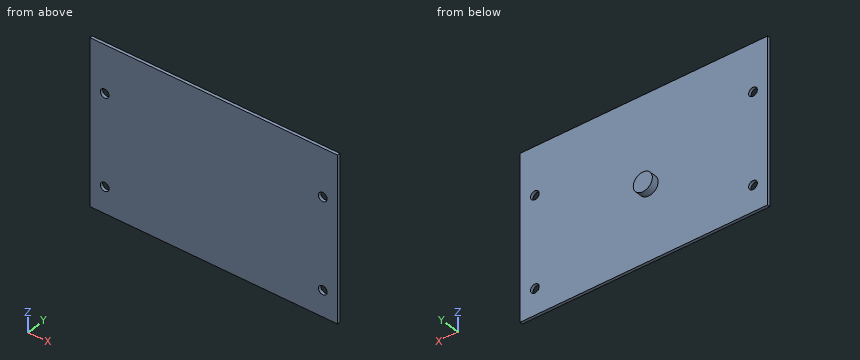
```python
from build123d import *

# Parameters (mm, degrees)
SKETCH1_W           = 85.09
SKETCH1_H           = 56.134
SKETCH1_R           = 1.5
BOSS_EXTRUDE1_DEPTH = 1
SKETCH2_R           = 3.283223987
BOSS_EXTRUDE2_DEPTH = 2.5


with BuildPart() as part:
    # Sketch1 → Boss-Extrude1 (new body)
    with BuildSketch(Plane(origin=(0, 0, 0), x_dir=(1, 0, 0), z_dir=(0, 1, 0))):
        with Locations((42.545, 28.067)):
            Rectangle(SKETCH1_W, SKETCH1_H)
        with Locations(Location((5.01, 47.244, 0), (0, 0, 270))):
            Circle(SKETCH1_R, mode=Mode.SUBTRACT)
        with Locations(Location((80.01, 47.244, 0), (0, 0, 270))):
            Circle(SKETCH1_R, mode=Mode.SUBTRACT)
        with Locations(Location((5.01, 16.244, 0), (0, 0, 270))):
            Circle(SKETCH1_R, mode=Mode.SUBTRACT)
        with Locations(Location((80.01, 16.244, 0), (0, 0, 270))):
            Circle(SKETCH1_R, mode=Mode.SUBTRACT)
    extrude(amount=BOSS_EXTRUDE1_DEPTH)

    # Sketch2 → Boss-Extrude2 (add)
    with BuildSketch(Plane(origin=(0, 1, 0), x_dir=(1, 0, 0), z_dir=(0, 1, 0))):
        with Locations(Location((40.898145706, 31.154537448, 0), (0, 0, 90))):
            Circle(SKETCH2_R)
    extrude(amount=BOSS_EXTRUDE2_DEPTH)


solid = part.part
```
Input: part model. Units: mm. Frame: model coordinates. Coordinates: 2 decimals unless noted, no trailing zeros. Order: outer loops, then holes, each group sorted by start corner. A loop starts at its lowest first (then second) coordinate and runs counter-clockwise, first axis right, second up. Notation, with made-up numbers: (-5, 47.25) - (-1, 47.25) arc R15 cw to (-1, 62.25) - close; hole circle Ø1 at (-13, 35). An arc over 180 degrees is marked (long way). Return JSON: item names as keys, results as strings.
Q1. Ray query, probe 1 along Z at (x, y) = (80.01, 0.45); probe 2 along Z at (x, y) = (6, 0.5); probe 3 along Y at (x, z) = (25, -48). Return the intervals inside material, ascending.
The answers:
{"probe 1": "z = -56.13 to -48.74, -45.74 to -17.74, -14.74 to 0", "probe 2": "z = -56.13 to -48.37, -46.12 to -17.37, -15.12 to 0", "probe 3": "y = 0 to 1"}
Q2. Cut plane A-A (x = 5.01). Return loops of the section in (y, z).
The answers:
{"outline": "(0, -56.13) - (1, -56.13) - (1, -48.74) - (0, -48.74) - close; (0, -45.74) - (1, -45.74) - (1, -17.74) - (0, -17.74) - close; (0, -14.74) - (1, -14.74) - (1, 0) - (0, 0) - close"}
Q3. Cut plane D-D (y = 1.95). Return loops of the section in (x, z).
The answers:
{"outline": "circle Ø6.57 at (40.9, -31.15)"}
Q4. First-contact query: pin 1 (4 mm diameter, centred on x = 5.01, z = -47.244, fed in from +Y). Flat tip, straight axial feed; report the tip coordinate or a pass-through.
The answers:
{"pin 1": "stops at y = 1"}
Q5. Cut plane B-B (z = -32.5). Return loops of the section in (x, y), then the cut area to 3 significant figures.
The answers:
{"outline": "(0, 0) - (85.09, 0) - (85.09, 1) - (43.89, 1) - (43.89, 3.5) - (37.9, 3.5) - (37.9, 1) - (0, 1) - close", "area": "100 mm2"}
Q6. Cut plane C-C (x = 39.5). Return loops of the section in (y, z), then the cut area to 3 significant figures.
The answers:
{"outline": "(0, -56.13) - (1, -56.13) - (1, -34.13) - (3.5, -34.13) - (3.5, -28.18) - (1, -28.18) - (1, 0) - (0, 0) - close", "area": "71.0 mm2"}
